The figure shows three views and two pictorial views of one solid part (mm, origin at its lowest corner). Answer the questions. Give positions to 0.01 mm unless a question says otherwise; leave off trailing zeros. Loops run counter-clockwise (first coordinate to the right, second up) from the corner with the lowest first, then second, coordinate; pieces in that order, holes last. Notation, with made-up numbers: (-6, 44.5) - (14, 44.5) arc R22 cw to (14, 57.5) - close; hole circle Ø7 at (30.5, 16). An arc over 180 degrees is marked (long way). Write each question's results on one line, items separated by ' | '.
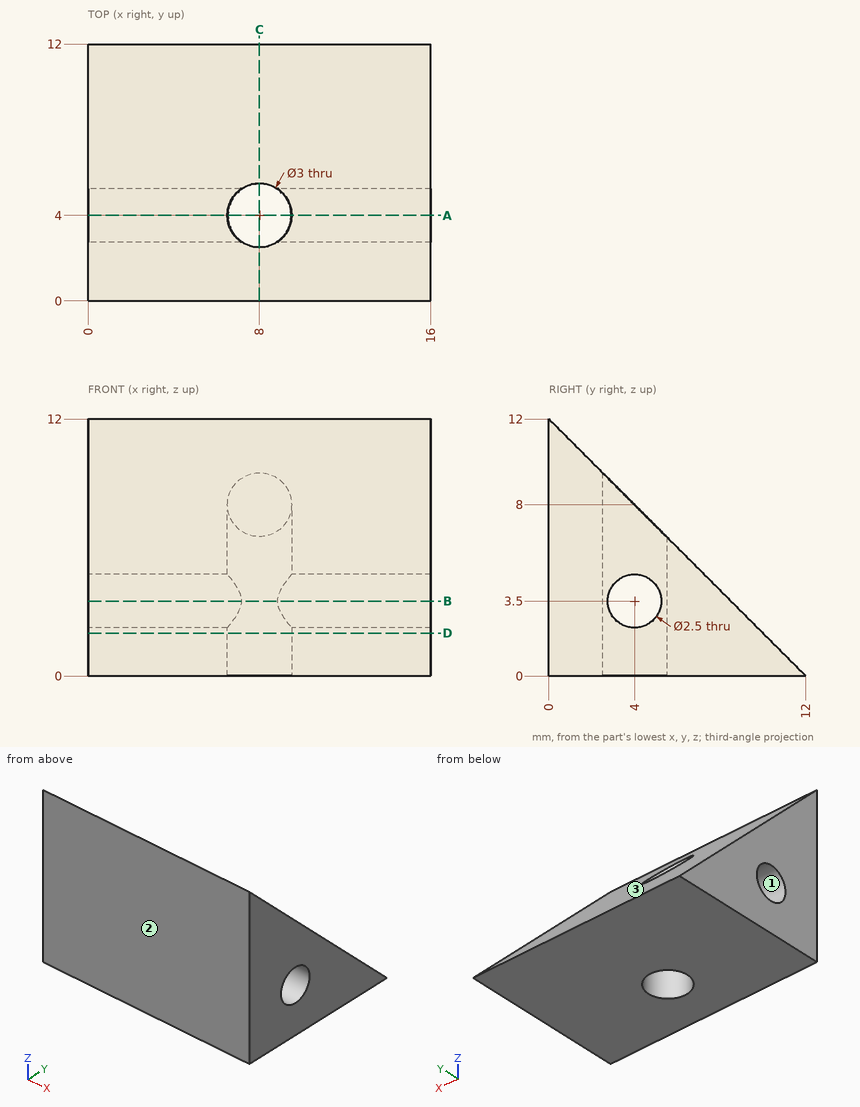
Item 1: A cutting plane is placed at B-B, the plane z = 3.5. Determine the outline of the cut face in (x, y), plus the area to 3 significant figures.
Values found:
outline: (0, 0) - (16, 0) - (16, 2.75) - (8.83, 2.75) arc R1.5 cw to (7.17, 2.75) - (0, 2.75) - close; (0, 5.25) - (7.17, 5.25) arc R1.5 cw to (8.83, 5.25) - (16, 5.25) - (16, 8.5) - (0, 8.5) - close | area: 95.4 mm²
Item 2: Flat-ended cylindrical pins translate along their axes: P1, Ø6, axis at y = 8, z = 4.5, coming from the -X side; P2, Ø5, axis at x = 9, y = 8, coming from the +Z side; P3, Ø1, axis at x = 9.5, y = 6.5, coming from the +Z side; P4, Ø4, axis at x = 8, y = 4, coming from the +Z side. Find the tip coordinate at first contact, or state that the pin passes through.
Values found:
P1: stops at x = 0 | P2: stops at z = 6.5 | P3: stops at z = 6 | P4: stops at z = 10
Item 3: A cutting plane is placed at D-D, the plane z = 2. Determine the outline of the cut face in (x, y).
Values found:
outline: (0, 0) - (16, 0) - (16, 10) - (0, 10) - close; hole circle Ø3 at (8, 4)
Item 4: Find the intervals of material crossed by line 1 along X through (y, z) = (2.75, 1); line 2 along Y through (x, z) = (12.5, 3.5); line 3 along Z through (x, y) = (5, 6.5), in increasing order. Write a range as [from, to].
Values found:
line 1: x = [0, 7.17], [8.83, 16] | line 2: y = [0, 2.75], [5.25, 8.5] | line 3: z = [0, 5.5]
Item 5: A cutting plane is placed at A-A, the plane y = 4. Determine the outline of the cut face in (x, z).
Values found:
outline: (0, 0) - (6.5, 0) - (6.5, 2.25) - (0, 2.25) - close; (0, 4.75) - (6.5, 4.75) - (6.5, 8) - (0, 8) - close; (9.5, 0) - (16, 0) - (16, 2.25) - (9.5, 2.25) - close; (9.5, 4.75) - (16, 4.75) - (16, 8) - (9.5, 8) - close
Item 6: A cutting plane is placed at C-C, the plane x = 8. Determine the outline of the cut face in (y, z), plus the area to 3 significant figures.
Values found:
outline: (0, 0) - (2.5, 0) - (2.5, 9.5) - (0, 12) - close; (5.5, 0) - (12, 0) - (5.5, 6.5) - close | area: 48.0 mm²
Item 7: For a pull along Y with two mould halves and no side action, classify the marked faces 1, 2 and 3 as released by +Y, released by -Y, zero draft, split by the parting line, or undercut.
Values found:
face 1: undercut | face 2: released by -Y | face 3: released by +Y
